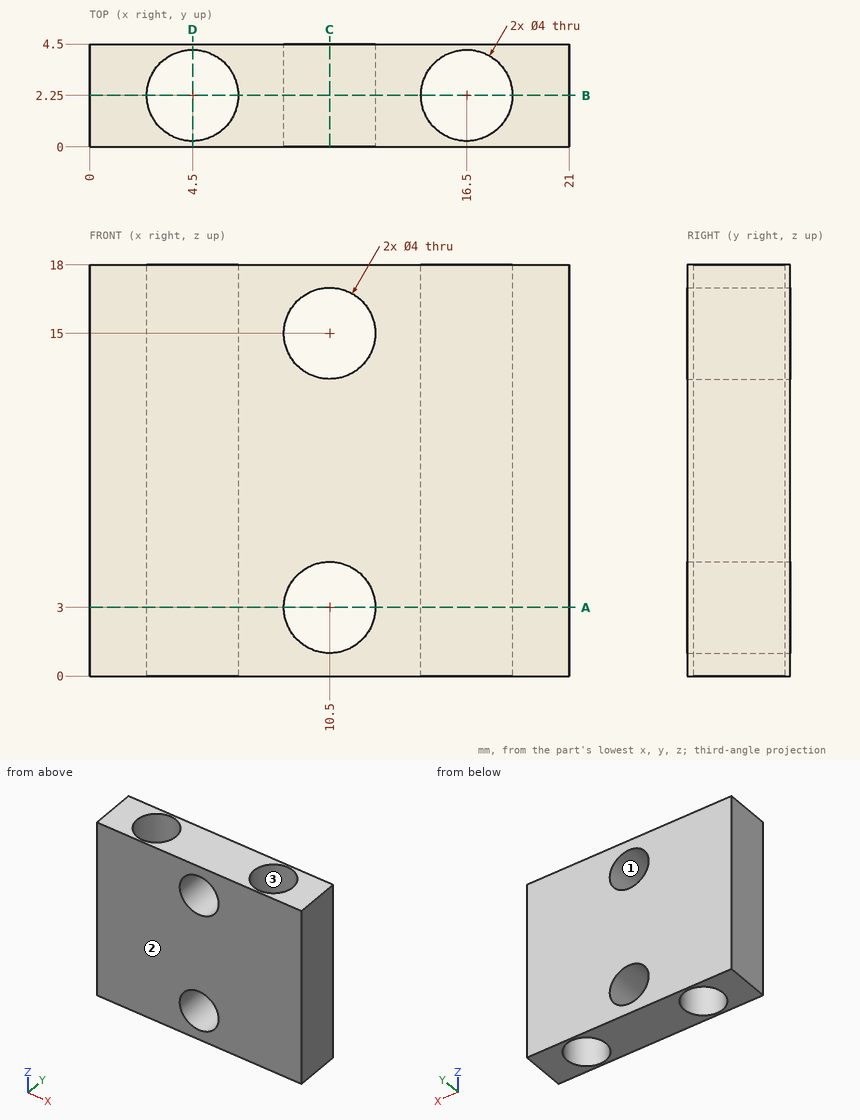
Answer from the drawing. Dimensions are ordinates in mm from the lowest x, y and z of the part. Give positions to 0.01 mm unless a question says otherwise; leave off trailing zeros. Order: outer loops, then holes, each group sorted by start corner. A loop starts at its lowest first (then second) coordinate and runs counter-clockwise, first axis right, second up. Notation, with made-up numbers: (-19, 17.25) - (32, 17.25) arc R33 ccw to (32, 54.25) - close; hole circle Ø11 at (-23, -5). An arc over 180 degrees is marked (long way). One line per item, written item: value. Start each with the question number.
1. Section B-B, the plane y = 2.25 is taken. Write down the section's boundary in (x, z), then the cut area to 3 significant figures.
2. Consider line 1 (X direction, y = 2.15, z = 15); line 2 (Z direction, x = 10.5, y = 3.4); line 3 (Z direction, x = 11.25, y = 4.1). Determine where each line is inside the solid, lowest interval first.
3. Section C-C, the plane x = 10.5 is taken. Write down the section's boundary in (y, z).
4. Section A-A, the plane z = 3 is taken. Write down the section's boundary in (x, y).
5. For a pull along Y with two mould halves and no side action, classify the marked faces 1, 2 and 3 as released by +Y, released by -Y, zero draft, split by the parting line, or undercut.
6. Each of these flat-tipped pins is pushed along its axis until it touches: pin 1 Ø4.5 at (x, z) = (10.5, 15) entering from -Y; pin 2 Ø3.5 at (x, z) = (10.5, 3) entering from -Y. Where does it stop, or does it pass through?
7. Section D-D, the plane x = 4.5 is taken. Write down the section's boundary in (y, z), then the cut area to 3 significant figures.
Filled sheet:
1. outline: (0, 0) - (2.5, 0) - (2.5, 18) - (0, 18) - close; (6.5, 0) - (14.5, 0) - (14.5, 18) - (6.5, 18) - close; (18.5, 0) - (21, 0) - (21, 18) - (18.5, 18) - close; hole circle Ø4 at (10.5, 3); hole circle Ø4 at (10.5, 15)
1. area: 209 mm²
2. line 1: 0 to 2.5, 6.5 to 8.5, 12.5 to 14.5, 18.5 to 21
2. line 2: 0 to 1, 5 to 13, 17 to 18
2. line 3: 0 to 1.15, 4.85 to 13.15, 16.85 to 18
3. outline: (0, 0) - (4.5, 0) - (4.5, 1) - (0, 1) - close; (0, 5) - (4.5, 5) - (4.5, 13) - (0, 13) - close; (0, 17) - (4.5, 17) - (4.5, 18) - (0, 18) - close
4. outline: (0, 0) - (8.5, 0) - (8.5, 4.5) - (0, 4.5) - close; (12.5, 0) - (21, 0) - (21, 4.5) - (12.5, 4.5) - close; hole circle Ø4 at (4.5, 2.25); hole circle Ø4 at (16.5, 2.25)
5. face 1: zero draft
5. face 2: released by -Y
5. face 3: undercut
6. pin 1: y = 0
6. pin 2: through
7. outline: (0, 0) - (0.25, 0) - (0.25, 18) - (0, 18) - close; (4.25, 0) - (4.5, 0) - (4.5, 18) - (4.25, 18) - close
7. area: 9.00 mm²
